from build123d import *

# Parameters (mm, degrees)
F0_W     = 8.5
F0_H     = 3.7
F1_DEPTH = 1.75
F2_W     = 0.5
F2_H     = 0.3
F3_DEPTH = 3.7
F4_W     = 2
F4_H     = 1.5
F5_DEPTH = 0.2
F4_W_2   = 1.5
F6_DEPTH = 4


with BuildPart() as f1:
    # F0 (on Front) → F1 (new body, symmetric)
    with BuildSketch(Plane.XZ):
        Rectangle(F0_W, F0_H)
    extrude(amount=F1_DEPTH, both=True)

    # F2 (on face) → F3 (join)
    with BuildSketch(Plane(origin=(0, 1.75, 0), x_dir=(-1, 0, 0), z_dir=(0, 1, 0))):
        Rectangle(F2_W, F2_H)
        with Locations((2.5, 0)):
            Rectangle(F2_W, F2_H)
        with Locations((-2.5, 0)):
            Rectangle(F2_W, F2_H)
    extrude(amount=F3_DEPTH)

    # F4 (on face) → F5 (cut)
    with BuildSketch(Plane.XZ.offset(1.75)):
        with Locations((0.75, 0)):
            Rectangle(F4_W, F4_H)
    extrude(amount=-F5_DEPTH, mode=Mode.SUBTRACT)

    # F4 (on face) → F6 (join)
    with BuildSketch(Plane.XZ.offset(1.75)):
        with Locations((-1, 0)):
            Rectangle(F4_W_2, F4_H)
    extrude(amount=F6_DEPTH)


solid = f1.part
Could you check a few things on this model? Use its own coordinates, in mm. A direction names the side the tool comes from. Coordinates: 2 decimals unless noted, no trailing zeros. Loops run counter-clockwise (first coordinate to the right, second up) from the corner with the lowest first, then second, coordinate; pieces in that order, holes last.
1. We'd pull the mould along X, two halves only. Please class faces 1 (the face through (1, -1.55, 0)), 2 (the face through (-4.25, 0, 0)), 3 (the face through (4.25, 0, 0)), 4 (the face through (-1, -4, 0.75)): released by +X, released by -X, zero draft, split by the parting line, or undercut.
2. I need wall thicknesses on L1, parallel to Y at x = -3.25, z = 0.3; L2, parallel to X at y = -2, z = 0.3; L3, parallel to Y at x = 1.5, z = -0.15. Which ranges of each line are inside material? Lowest first, please.
3. Imagine slicing it at A-A (y = 5). Please give me the cut outline in (x, z), and give its area (3 significant figures).
4. Imagine slicing it at B-B (x = 2.5). Please give me the cut outline in (y, z), and give its area (3 significant figures).
5. For P1, Ø0.8, axis at y = -4.5, z = 0, coming from the -X side; P2, Ø0.8, axis at x = 0.5, z = 0, coming from the -Y side; P3, Ø0.6, axis at x = -2.5, y = 3.5, coming from the -Z side, each with a flat end and sliding along its axis, tell me the tip position at first contact or that it passes through.
6. For faces 5 (the face through (-1, -4, -0.75)), 6 (the face through (-1.75, -4, 0)), 7 (the face through (0, 0, -1.85)), which set-ups out of +Z, -Z, +X, -X, +Y, -Y let a thin tool reach every point of the face, with its end or its side?
7. Imagine slicing it at C-C (z = 0.9). Please give me the cut outline in (x, y), and give its area (4 significant figures).
8. Imagine slicing it at D-D (y = -2.5). Please give me the cut outline in (x, z), and give its area (3 significant figures).
Computed values:
1. face 1: undercut
1. face 2: released by -X
1. face 3: released by +X
1. face 4: zero draft
2. L1: y = -1.75 to 1.75
2. L2: x = -1.75 to -0.25
2. L3: y = -1.55 to 1.75
3. outline: (-2.75, -0.15) - (-2.25, -0.15) - (-2.25, 0.15) - (-2.75, 0.15) - close; (-0.25, -0.15) - (0.25, -0.15) - (0.25, 0.15) - (-0.25, 0.15) - close; (2.25, -0.15) - (2.75, -0.15) - (2.75, 0.15) - (2.25, 0.15) - close
3. area: 0.450 mm2
4. outline: (-1.75, -1.85) - (1.75, -1.85) - (1.75, -0.15) - (5.45, -0.15) - (5.45, 0.15) - (1.75, 0.15) - (1.75, 1.85) - (-1.75, 1.85) - close
4. area: 14.1 mm2
5. P1: stops at x = -1.75
5. P2: stops at y = -1.55
5. P3: stops at z = -0.15
6. face 5: -Z, +X, -X, -Y
6. face 6: +Z, -Z, -X, -Y
6. face 7: -Z, +X, -X, +Y, -Y
7. outline: (-4.25, -1.75) - (4.25, -1.75) - (4.25, 1.75) - (-4.25, 1.75) - close
7. area: 29.75 mm2
8. outline: (-1.75, -0.75) - (-0.25, -0.75) - (-0.25, 0.75) - (-1.75, 0.75) - close
8. area: 2.25 mm2
